```python
from build123d import *

# Parameters (mm, degrees)
EXTRUDE_1_DEPTH     = 5.5
SKETCH_2_R          = 2.1
CUT_EXTRUDE_2_DEPTH = 3
SKETCH_4_R          = 1.35
CUT_EXTRUDE_3_DEPTH = 7
FILLET_2_R          = 1
CHAMFER_1_SIZE      = 0.2


with BuildPart() as part:
    # 草图1 → 凸台-拉伸1 (new body)
    with BuildSketch(Plane(origin=(0, 0, 0), x_dir=(1, 0, 0), z_dir=(0, 1, 0))):
        with BuildLine():
            Line((-15, 25.980762114), (-12.5, 21.650635095))
            ThreePointArc((-12.5, 21.650635095), (0, 25), (12.5, 21.650635095))
            Line((12.5, 21.650635095), (15, 25.980762114))
            ThreePointArc((15, 25.980762114), (0, 30), (-15, 25.980762114))
        make_face()
    extrude(amount=EXTRUDE_1_DEPTH)

    # 草图2 → 切除-拉伸2 (cut)
    with BuildSketch(Plane(origin=(0, 5.5, 0), x_dir=(1, 0, 0), z_dir=(0, 1, 0))):
        with Locations(Location((-10.52379439, 25.406687144, 0), (0, 0, 270))):
            Circle(SKETCH_2_R)
        with Locations(Location((10.52379439, 25.406687144, 0), (0, 0, 270))):
            Circle(SKETCH_2_R)
    extrude(amount=-CUT_EXTRUDE_2_DEPTH, mode=Mode.SUBTRACT)

    # 草图4 → 切除-拉伸3 (cut)
    with BuildSketch(Plane(origin=(0, 5.5, 0), x_dir=(1, 0, 0), z_dir=(0, 1, 0))):
        with Locations(Location((-10.52379439, 25.406687144, 0), (0, 0, 270))):
            Circle(SKETCH_4_R)
        with Locations(Location((10.52379439, 25.406687144, 0), (0, 0, 270))):
            Circle(SKETCH_4_R)
    extrude(amount=-CUT_EXTRUDE_3_DEPTH, mode=Mode.SUBTRACT)

    # 圆角2
    fillet_2_edges = [part.edges().sort_by_distance(p)[0] for p in [
        (15, 2.75, -25.980762114),
        (12.5, 2.75, -21.650635095),
        (-12.5, 2.75, -21.650635095),
        (-15, 2.75, -25.980762114),
    ]]
    fillet(fillet_2_edges, radius=FILLET_2_R)

    # 倒角1
    chamfer_1_edges = [part.edges().sort_by_distance(p)[0] for p in [
        (0, 5.5, -30),
        (13.740878901, 5.5, -23.799900398),
        (-13.740878901, 5.5, -23.799900398),
        (0, 5.5, -25),
        (-12.401705751, 5.5, -22.039231077),
        (-14.586670486, 5.5, -25.875237728),
        (12.401705751, 5.5, -22.039231077),
        (14.586670486, 5.5, -25.875237728),
    ]]
    chamfer(chamfer_1_edges, length=CHAMFER_1_SIZE)


solid = part.part
```
The model under review builds one solid part; all positions refer to its coordinate system, in mm. A direction names the side the tool comes from. Round coordinates to 2 decimals unless told otherwise and drop trailing zeros. Order: outer loops, then holes, each group sorted by start corner. A loop starts at its lowest first (then second) coordinate and runs counter-clockwise, first axis right, second up. Notation, with made-up numbers: (-8.75, 9) -> (12.25, 9) arc R26 ccw to (12.25, 27) -> close; hole circle Ø5 at (75, 1). An arc over 180 degrees is marked (long way). One line per item, written item: value. Start each with the question number.
Q1. Clearance check with flat-ended pins moving along their axes: pin 1 Ø4.5 at (x, z) = (9.5, -25) entering from +Y; pin 2 Ø1 at (y, z) = (1, -27) entering from +X; pin 3 Ø3 at (x, y) = (2, 4) entering from -Z; pin 4 Ø1.6 at (x, z) = (10.52, -25.41) entering from -Y. State where each tip first meets the part, or that it passes through.
Q2. Mouldability with a two-part tool opening along X and no side actions: class faces 1 (the face through (9, 2.5, -25)), 2 (the face through (-13.751, 2.613, -23.818)), 3 (the face through (13.73, 2.61, -23.78)), 4 (the face through (0, 3, -25)) as released by +X, released by -X, zero draft, split by the parting line, or undercut.
Q3. Take a section at B-B (y = 1.5). Write out the cut boundary in (x, z).
Q4. Machinability: for faces 5 (the face through (11.155, 4.021, -23.404)), 6 (the face through (0, 3, -30)), which of the approach directions +Z, -Z, +X, -X, +Y, -Y give a long, thin tool a straight path to every point of the face, cutting with its end or side? Answer none if there is none.
Q5. Take a section at D-D (y = 4.1). Write out the cut boundary in (x, z), and give its area (3 significant figures).
Q6. Wall thickness on line 1 (X direction, y = 4.5, z = -26.25); line 2 (Z direction, x = -11.5, y = 0.55); line 3 (X direction, y = 1.85, z = -26.5): over which ranges is each line inside the solid? List them lowest first.
Q7. Take a section at A-A (x = 0). Write out the cut boundary in (y, z), and give its area (3 significant figures).
Q8. Take a section at C-C (z = -25.5). Count the separate pieces of the cut face and the enclosed holes in it, and give its area (3 significant figures).
Reported:
1. pin 1: stops at y = 5.5
1. pin 2: stops at x = 14.06
1. pin 3: stops at z = -30
1. pin 4: passes through
2. face 1: undercut
2. face 2: released by -X
2. face 3: released by +X
2. face 4: undercut
3. outline: (-14.49, -25.1) arc R1 ccw to (-14.1, -26.48) arc R30 ccw to (14.1, -26.48) arc R1 ccw to (14.49, -25.1) -> (12.99, -22.5) arc R1 ccw to (11.66, -22.12) arc R25 cw to (-11.66, -22.12) arc R1 ccw to (-12.99, -22.5) -> close; hole circle Ø2.7 at (-10.52, -25.41); hole circle Ø2.7 at (10.52, -25.41)
4. face 5: +Y
4. face 6: -Z, +Y, -Y
5. outline: (-14.49, -25.1) arc R1 ccw to (-14.1, -26.48) arc R30 ccw to (14.1, -26.48) arc R1 ccw to (14.49, -25.1) -> (12.99, -22.5) arc R1 ccw to (11.66, -22.12) arc R25 cw to (-11.66, -22.12) arc R1 ccw to (-12.99, -22.5) -> close; hole circle Ø4.2 at (-10.52, -25.41); hole circle Ø4.2 at (10.52, -25.41)
5. area: 115 mm2
6. line 1: x = -14.39 to -12.45, -8.6 to 8.6, 12.45 to 14.39
6. line 2: z = -27.71 to -26.34, -24.47 to -22.2
6. line 3: x = -14.06 to -11.32, -9.73 to 9.73, 11.32 to 14.06
7. outline: (0, -30) -> (5.3, -30) -> (5.5, -29.8) -> (5.5, -25.2) -> (5.3, -25) -> (0, -25) -> close
7. area: 27.5 mm2
8. separate pieces: 3
8. enclosed holes: 0
8. area: 122 mm2
